Print and shaded views of the part. All mm, measured from the part's lowest x, y and z. A direction names the side the tool comes from. Round coordinates to 2 decimals unless told otherwise and drop trailing zeros. Loops run counter-clockwise (first coordinate to the right, second up) from the corner with the lowest first, then second, coordinate; pieces in that order, holes last. Notation, with made-up numbers: (28.25, 57.5) -> (62.25, 57.5) arc R25 cw to (62.25, 76.5) -> close; hole circle Ø2 at (-19, 10). An arc over 180 degrees is marked (long way). Answer as CSV lines item,"result".
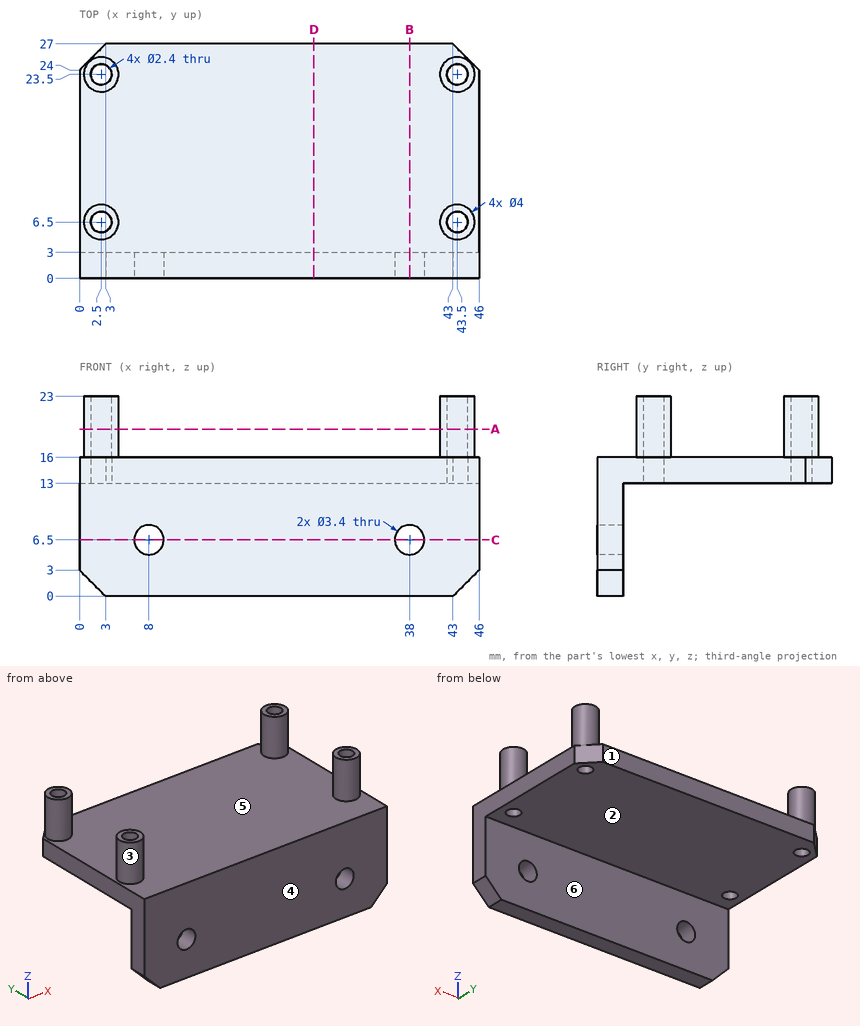
Q1. Drop flat-ended pins along their axis: pin 1 Ø12 at (x, z) = (21, 3.5) entering from +Y; pin 2 Ø10 at (x, y) = (31, 9.5) entering from -Z; pin 3 Ø12 at (x, y) = (40, 14) entering from +Z. Give the stop position or say it passes through.
Results:
pin 1,"y = 3"
pin 2,"z = 13"
pin 3,"z = 16"
Q2. Slice it at D-D, the plane x = 27. Give the cut face in (y, z), and give its area (3 significant figures).
Results:
outline,"(0, 0) -> (3, 0) -> (3, 13) -> (27, 13) -> (27, 16) -> (0, 16) -> close"
area,"120 mm2"
Q3. Slice it at A-A, the plane z = 19.25. Give the cut face in (x, y), and give its area (3 significant figures).
Results:
outline,"circle Ø4 at (2.5, 6.5); circle Ø4 at (2.5, 23.5); circle Ø4 at (43.5, 6.5); circle Ø4 at (43.5, 23.5); hole circle Ø2.4 at (2.5, 6.5); hole circle Ø2.4 at (2.5, 23.5); hole circle Ø2.4 at (43.5, 6.5); hole circle Ø2.4 at (43.5, 23.5)"
area,"32.2 mm2"
Q4. Two-plate mould, pull along Y, no slides. Class the marked faces 1, 2 and 3: pulls with the +Y half, pulls with the -Y half, needs draft (parallel to the pull), parting line crosses it, or undercut.
Results:
face 1,"pulls with the +Y half"
face 2,"needs draft"
face 3,"undercut"
Q5. Slice it at C-C, the plane z = 6.5. Give the cut face in (x, y).
Results:
outline,"(0, 0) -> (6.3, 0) -> (6.3, 3) -> (0, 3) -> close; (9.7, 0) -> (36.3, 0) -> (36.3, 3) -> (9.7, 3) -> close; (39.7, 0) -> (46, 0) -> (46, 3) -> (39.7, 3) -> close"
Q6. Probe L1, parallel to Y at x = 2.5, z = 18.5; L2, parallel to X at y = 2.4, z = 6.5; L3, parallel to X at y = 6.5, z = 15.5. List the from-to ranges inside material, lowest first. Write a range as [from, to].
Results:
L1,"[4.5, 5.3], [7.7, 8.5], [21.5, 22.3], [24.7, 25.5]"
L2,"[0, 6.3], [9.7, 36.3], [39.7, 46]"
L3,"[0, 1.3], [3.7, 42.3], [44.7, 46]"
Q7. Slice it at B-B, the plane x = 38. Give the cut face in (y, z).
Results:
outline,"(0, 0) -> (3, 0) -> (3, 4.8) -> (0, 4.8) -> close; (0, 8.2) -> (3, 8.2) -> (3, 13) -> (27, 13) -> (27, 16) -> (0, 16) -> close"
Q8. Tool access for the marked faces 4, 5 and 6: list every direction of +Z, -Z, +X, -X, +Y, -Y with a clear straight run to the whole face (end or side of a thin tool).
Results:
face 4,"+Z, -Z, +X, -X, -Y"
face 5,"+Z"
face 6,"-Z, +X, -X, +Y"
